```python
from build123d import *

# Parameters (mm, degrees)
F0_W     = 117.271182
F0_H     = 109.656172
F2_DEPTH = 71.374
F1_R     = 6.663407


with BuildPart() as f2:
    # F0 (on Top) → F2 (new body)
    with BuildSketch(Plane.XY):
        Rectangle(F0_W, F0_H)
    extrude(amount=-F2_DEPTH)

    # F1 (on Top) → F4 (revolve)
    with BuildSketch(Plane.XY):
        with Locations((39.96164, 0)):
            Circle(F1_R)
    revolve(axis=Axis((0, -0.142617, 0), (0, -1, 0)))


solid = f2.part
```
Input: part model. Units: mm. Frame: model coordinates. Round coordinates to 2 decimals unless told otherwise and drop trailing zeros. Write each loop counter-clockwise with the first axis right and the second up, starting at its lowest first coordinate (ties: lowest second). Pieces come first, ordered by that corner, then holes. Notation, with made-up numbers: (-12.75, 24.5) -> (26.25, 24.5) arc R22 ccw to (26.25, 43.5) -> close; hole circle Ø6 at (49.25, 80.5). An arc over 180 degrees is marked (long way). Answer as CSV lines item,"result".
1. Ray query, L1, parallel to Z at x = 16.5, y = -20; L2, parallel to Z at x = 12, y = -1.5; L3, parallel to Y at x = 32.5, z = 26.5. Return the intervals inside material, ascending. Write a range as [from, to].
Geometry says:
L1,"z = [-71.37, 0]"
L2,"z = [-71.37, 0], [31.24, 44.88]"
L3,"y = [-6.36, 6.36]"
2. Section A-A (y = 5). Return the cut outline in (x, z), plus the area to 3 significant figures.
Geometry says:
outline,"(-58.64, -71.37) -> (58.64, -71.37) -> (58.64, 0) -> (44.37, 0) arc R44.37 ccw to (-44.37, 0) -> (-58.64, 0) -> close; hole (-35.56, 0) -> (35.56, 0) arc R35.56 ccw to start"
area,"9,480 mm^2"
3. Section B-B (y = -19.5). Return the cut outline in (x, z), plus the area to 3 significant figures.
Geometry says:
outline,"(-58.64, -71.37) -> (58.64, -71.37) -> (58.64, 0) -> (-58.64, 0) -> close"
area,"8,370 mm^2"
4. Contact query for a flat-ended pin moving along its axis: P1, Ø3, axis at x = -5, y = -3.5, coming from the +Z side. Output: stop coordinate, or through.
Geometry says:
P1,"stops at z = 46.07"
